Model file for the job. Use its own axes, mm. Round coordinates to 2 decimals unless told otherwise and drop trailing zeros. Loops run counter-clockwise (first coordinate to the right, second up) from the corner with the lowest first, then second, coordinate; pieces in that order, holes last. Notation, with made-up numbers: (-8, 28) - (1, 28) arc R15 ccw to (1, 43) - close; hole circle Ø5 at (64, 65.5). An arc over 180 degrees is marked (long way). Use one line per item in the form item = value.
Autodesk Fusion 360 part; units mm, degrees
sketch "Sketch1" plane through (0, 0, 0) normal (0, 0, 1) x (1, 0, 0)
  line L0 (36.0554, 51.2556) -> (91.0554, 51.2556)
  line L1 (91.0554, 51.2556) -> (91.0554, 10.2556)
  line L2 (36.0554, 10.2556) -> (36.0554, 51.2556)
  line L3 (33.0554, 13.2556) -> (33.0554, 54.2556)
  line L4 (33.0554, 54.2556) -> (94.0554, 54.2556)
  line L5 (36.0554, 10.2556) -> (18.0554, 10.2556)
  line L6 (18.0554, 10.2556) -> (18.0554, 13.2556)
  line L7 (18.0554, 13.2556) -> (33.0554, 13.2556)
  line L8 (91.0554, 10.2556) -> (109.0554, 10.2556)
  line L9 (109.0554, 10.2556) -> (109.0554, 13.2556)
  line L10 (109.0554, 13.2556) -> (94.0554, 13.2556)
  line L11 (94.0554, 54.2556) -> (94.0554, 13.2556)
  line L12 (33.0554, 13.2556) -> (36.0554, 13.2556)
  line L13 (94.0554, 13.2556) -> (91.0554, 13.2556)
  dimension "d1" = 55
  dimension "d2" = 41
  dimension "d4" = 18
  dimension "d5" = 3
  dimension "d6" = 18
  dimension "d7" = 3
extrude "Extrude3" add sketch "Sketch1" along normal blind 7.5 contours L2 L5 L6 L7 L12 | L1 L8 L9 L10 L13 makes body 1 at (30.0554, 10.2556, 2.5) makes body 2 at (103.0554, 13.2556, 2.5)
extrude "Extrude2" add sketch "Sketch1" along normal blind 5 separate body contours L0 L1 L2 L3 L4 L11 L12 L13 makes body 3
extrude "Extrude4" add sketch "Sketch1" against normal blind 2.5 contours L2 L5 L6 L7 L12 | L1 L8 L9 L10 L13 bodies 1 2 3
hole "Hole1" at (25.5554, 13.2556, 2.5) direction (0, -1, 0) diameter 5 depth 10 tip angle 118 countersink diameter 8 countersink angle 90 bodies 1
ref_plane "WorkPlane1" through (63.5554, 33.7556, 2.5) normal (-1, 0, 0) x (0, -1, 0)
mirror "Mirror1" about plane through (63.5554, 33.7556, 2.5) normal (-1, 0, 0) of "Hole1"
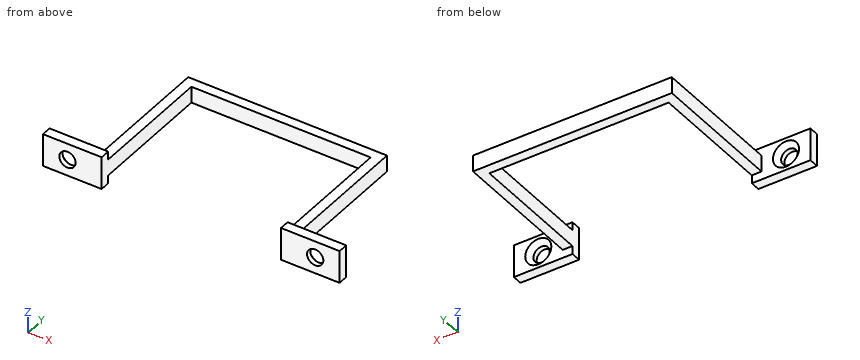
1. Cut at C-C, the plane x = 69.5. Give the cut face in (y, z).
Geometry check:
outline = (51.26, 0) - (54.26, 0) - (54.26, 5) - (51.26, 5) - close
2. Flat gauge pins, fed straight in: pin 1 (6 mm diameter, centred on x = 56.5, z = 6, fed in from +Y); pin 2 (5 mm diameter, centred on x = 96, y = 44, fed in from -Z); pin 3 (3 mm diameter, centred on y = 31.5, z = 2, fed in from +X); pin 4 (4 mm diameter, centred on y = 23.5, z = 2, fed in from -X). Where does each tip first touch, or does it go through?
Geometry check:
pin_1 = 54.26
pin_2 = 0
pin_3 = 94.06
pin_4 = 33.06
3. Wall check: probe 1 along X at (y, z) = (11.3, 2.5); probe 2 along X at (y, z) = (19, 1.5); probe 3 along Y at (x, z) = (79, 0.75). Give the ranges that are in metal, low to high.
Geometry check:
probe_1 = 18.06 to 23.06, 28.06 to 36.06, 91.06 to 99.06, 104.06 to 109.06
probe_2 = 33.06 to 36.06, 91.06 to 94.06
probe_3 = 51.26 to 54.26
4. Cut at A-A, the plane y = 41.5. Give the cut face in (x, z), plus the area to 3 significant figures.
Geometry check:
outline = (33.06, 0) - (36.06, 0) - (36.06, 5) - (33.06, 5) - close; (91.06, 0) - (94.06, 0) - (94.06, 5) - (91.06, 5) - close
area = 30.0 mm^2
5. Cut at B-B, the plane z = 2.5. Give the cut face in (x, y), plus the area to 4 significant figures.
Geometry check:
outline = (18.06, 10.26) - (23.06, 10.26) - (23.06, 11.76) - (21.56, 13.26) - (18.06, 13.26) - close; (28.06, 10.26) - (36.06, 10.26) - (36.06, 51.26) - (91.06, 51.26) - (91.06, 10.26) - (99.06, 10.26) - (99.06, 11.76) - (97.56, 13.26) - (94.06, 13.26) - (94.06, 54.26) - (33.06, 54.26) - (33.06, 13.26) - (29.56, 13.26) - (28.06, 11.76) - close; (104.06, 10.26) - (109.06, 10.26) - (109.06, 13.26) - (105.56, 13.26) - (104.06, 11.76) - close
area = 484.5 mm^2
